Could you check a few things on this drawing? It's one solid part, dimensions in mm from its lowest x, y, z. A direction names the side the tool comes from. Coordinates: 2 decimals unless noted, no trailing zeros. Write each loop counter-clockwise with the first axis right and the second up, starting at its lowest first coordinate (ties: lowest second). Pieces come first, ordered by that corner, then holes.
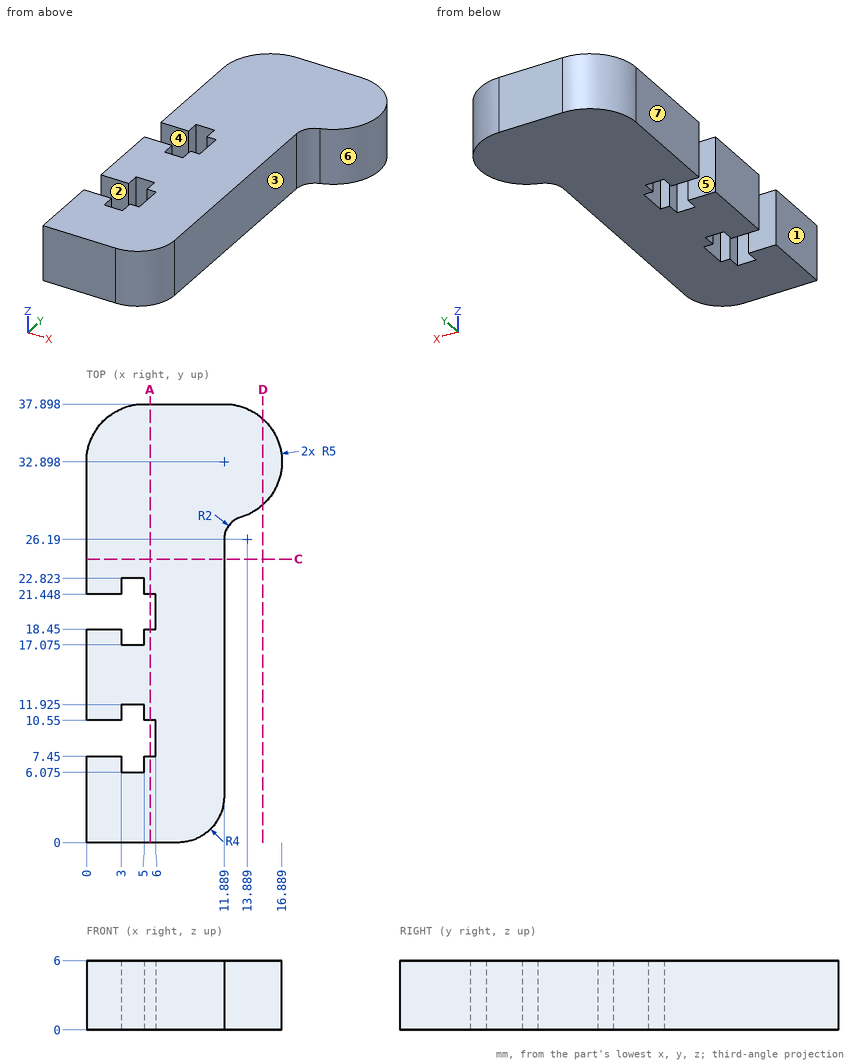
1) We'd pull the mould along Y, two halves only. Please class the marked faces 4, 5, 6 and 7: pulls with the +Y half, pulls with the -Y half, needs draft (parallel to the pull), parting line crosses it, or undercut.
Values follow:
face 4: undercut
face 5: undercut
face 6: parting line crosses it
face 7: needs draft
2) I need wall thicknesses on probe 1 along X at (y, z) = (11, 2.1); probe 2 along X at (y, z) = (24.5, 3.3); probe 3 along X at (y, z) = (33, 0.45). Which ranges of each line are inside material? Lowest first, please.
Values follow:
probe 1: x = 0 to 3, 5 to 11.89
probe 2: x = 0 to 11.89
probe 3: x = 0 to 16.89
3) Will these pins go through, and if not, where does the flat tip stop? pin 1 (10 mm diameter, centred on x = 4, y = 15.5, fed in from -Z); pin 2 (0.7 mm diameter, centred on y = 18, z = 4, fed in from +X); pin 3 (3.5 mm diameter, centred on x = 2, z = 3.5, fed in from +Y); pin 4 (0.9 mm diameter, centred on x = 1.5, z = 3.5, fed in from +Y).
Values follow:
pin 1: stops at z = 0
pin 2: stops at x = 11.89
pin 3: stops at y = 37.74
pin 4: stops at y = 36.86
4) Imagine slicing it at C-C on y = 24.5. Please give me the cut outline in (x, z).
Values follow:
outline: (0, 0) - (11.89, 0) - (11.89, 6) - (0, 6) - close
5) Imagine slicing it at A-A on x = 5.5. Please give me the cut outline in (y, z).
Values follow:
outline: (0, 0) - (7.45, 0) - (7.45, 6) - (0, 6) - close; (10.55, 0) - (18.45, 0) - (18.45, 6) - (10.55, 6) - close; (21.45, 0) - (37.9, 0) - (37.9, 6) - (21.45, 6) - close
6) Imagine slicing it at D-D on x = 15.25. Please give me the cut outline in (y, z).
Values follow:
outline: (29.2, 0) - (36.6, 0) - (36.6, 6) - (29.2, 6) - close
7) On a 3-axis mill with a long thin cutter (end or side, diameter ignored), from which of +Z, -Z, +X, -X, +Y, -Y can I reach the whole of each face in a straight line? I mean the marked faces 1, 2 and 3. Say none if no direction works.
Values follow:
face 1: +Z, -Z, -X, +Y, -Y
face 2: +Z, -Z, -X
face 3: +Z, -Z, +X, -Y
